Part model, mm, in its own coordinate system. Face numbers are marked on the shaded views. Round coordinates to 2 decimals unless told otherwise and drop trailing zeros. Write each loop counter-clockwise with the first axis right and the second up, starting at its lowest first coordinate (ties: lowest second). Pieces come first, ordered by that corner, then holes. Notation, with made-up numbers: (-20, 60.5) -> (29, 60.5) arc R22 cw to (29, 68.5) -> close; hole circle Ø5 at (54.5, 43). An arc over 180 degrees is marked (long way). Use CSV: the item, a comma, the result in double quotes. Start each with the question number.
(1) Saw through at D-D (z = 26). Give the cut face in (x, y), plus the area to 3 significant figures.
(2) Saw through at A-A (z = 82). Give the cut face in (x, y), plus the area to 3 significant figures.
(3) Drop flat-ended pins along their axis: pin 1 (2 mm diameter, centred on x = -12.5, y = -313, fed in from +Z); pin 2 (2.5 mm diameter, centred on x = -117, z = 5.5, fed in from -Y); pin 3 (8 mm diameter, centred on y = -860.5, z = 20.5, fed in from +X). Give the stop position or say it passes through.
(4) Probe line 1 (X direction, y = -360, z = 75.5); line 2 (X direction, y = -460.5, z = 68.5); line 3 (Z direction, x = -85.5, y = -888). List the from-to ranges inside material, lowest first. Write a range as [from, to].
(5) Saw through at C-C (x = 0). Give the cut face in (y, z), plus the area to 3 significant figures.
(6) Two-plate mould, pull along X, no slides. Class the marked faces 1 and 2: released by +X, released by -X, zero draft, split by the parting line, or undercut.
```python
from build123d import *

# Parameters (mm, degrees)
F1_DEPTH = 1219.2
F2_DEPTH = 101.6


with BuildPart() as f1:
    # F0 (on Front) → F1 (new body)
    with BuildSketch(Plane.XZ):
        with BuildLine():
            Line((101.592062, 1.27), (109.530137, 1.27))
            ThreePointArc((109.530137, 1.27), (109.406127, 5.363148), (109.129208, 9.4488))
            ThreePointArc((109.129208, 9.4488), (0, 109.5375), (-109.129208, 9.4488))
            ThreePointArc((-109.129208, 9.4488), (-109.406127, 5.363148), (-109.530137, 1.27))
            Line((-109.530137, 1.27), (-101.592062, 1.27))
            ThreePointArc((-101.592062, 1.27), (0, 101.6), (101.592062, 1.27))
        make_face()
    extrude(amount=F1_DEPTH)

    # F0 (on Front) → F2 (join)
    with BuildSketch(Plane.XZ):
        with BuildLine():
            Line((-139.692062, 1.27), (-127, 1.27))
            Line((-127, 1.27), (-109.530137, 1.27))
            ThreePointArc((-109.530137, 1.27), (-109.406127, 5.363148), (-109.129208, 9.4488))
            Line((-109.129208, 9.4488), (-139.692062, 9.4488))
            Line((-139.692062, 9.4488), (-139.692062, 1.27))
        make_face()
        with BuildLine():
            Line((109.530137, 1.27), (127, 1.27))
            Line((127, 1.27), (139.692062, 1.27))
            Line((139.692062, 1.27), (139.692062, 9.4488))
            Line((139.692062, 9.4488), (109.129208, 9.4488))
            ThreePointArc((109.129208, 9.4488), (109.406127, 5.363148), (109.530137, 1.27))
        make_face()
    extrude(amount=F2_DEPTH)


solid = f1.part
```
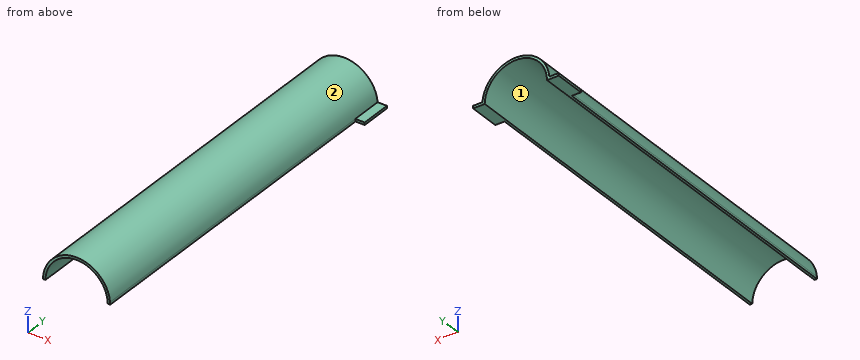
Answers:
1,outline,"(-106.41, -1219.2) -> (-98.22, -1219.2) -> (-98.22, 0) -> (-106.41, 0) -> close; (98.22, -1219.2) -> (106.41, -1219.2) -> (106.41, 0) -> (98.22, 0) -> close"
1,area,"20,000 mm²"
2,outline,"(-72.63, -1219.2) -> (-59.99, -1219.2) -> (-59.99, 0) -> (-72.63, 0) -> close; (59.99, -1219.2) -> (72.63, -1219.2) -> (72.63, 0) -> (59.99, 0) -> close"
2,area,"30,800 mm²"
3,pin 1,"stops at z = 108.93"
3,pin 2,"stops at y = -101.6"
3,pin 3,"stops at x = 108.29"
4,line 1,"x = [-79.36, -67.99], [67.99, 79.36]"
4,line 2,"x = [-85.48, -75.04], [75.04, 85.48]"
4,line 3,"z = [54.88, 68.47]"
5,outline,"(-1219.2, 101.6) -> (0, 101.6) -> (0, 109.54) -> (-1219.2, 109.54) -> close"
5,area,"9,680 mm²"
6,face 1,"undercut"
6,face 2,"split by the parting line"
